Here's the drawing with two shaded views (mm, measured from the low corner). I have some questions. A direction names the side the tool comes from. Round coordinates to 2 decimals unless told otherwise and drop trailing zeros. Loops run counter-clockwise (first coordinate to the right, second up) from the corner with the lowest first, then second, coordinate; pieces in that order, holes last.
(1) I want a section at A-A on z = 10. Write out the boundary of the cut face in (x, y).
(2) If I drill on line 1 along Z through (x, y) = (15, 1.6); line 2 along Z through (x, y) = (2.2, 15); line 3 along Y through (x, z) = (14.5, 1.25), over which ranges is the centre line in solid material (lowest first)?
(3) Thinking about a two-plate mould opening in Y: for the marked faces 1, 2 and 3, which applies, released by +Y, released by -Y, zero draft, split by the parting line, or undercut?
(4) Will these pins go through, and if not, where does the flat tip stop? pin 1 Ø5 at (x, z) = (14, 2.5) entering from +Y; pin 2 Ø5 at (y, z) = (26.5, 6) entering from +X.
(5) I want a section at C-C on y = 15. Write out the boundary of the cut face in (x, z).
(6) I want a section at B-B on x = 15. Write out the boundary of the cut face in (y, z), plus the area to 3 significant figures.
(7) I want a section at D-D on z = 2.75. Write out the boundary of the cut face in (x, y), plus the area to 3 significant figures.
(8) Which directions (+Z, -Z, +X, -X, +Y, -Y) give clear straight access to the entire face, cutting with the end or side of a thin tool? Please do the marked faces 4 and 5.
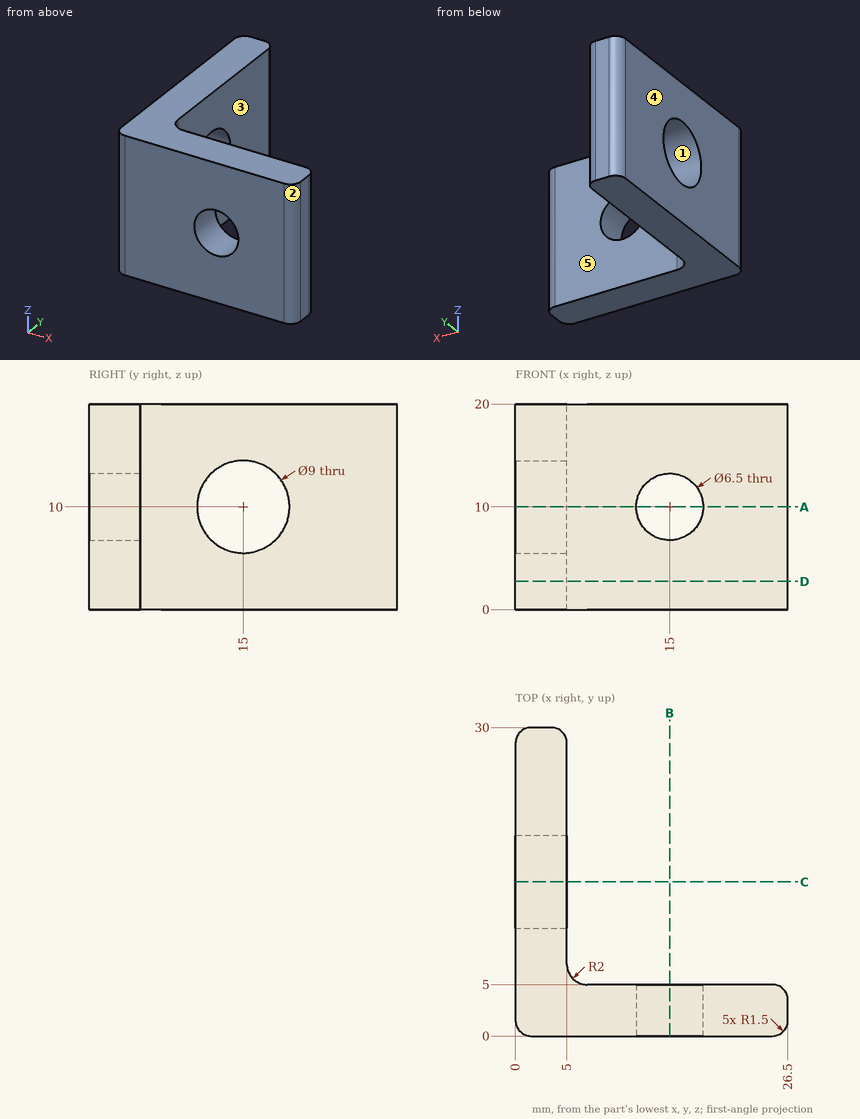
Filled sheet:
1. outline: (0, 1.5) arc R1.5 ccw to (1.5, 0) - (11.75, 0) - (11.75, 5) - (7, 5) arc R2 cw to (5, 7) - (5, 10.5) - (0, 10.5) - close; (0, 19.5) - (5, 19.5) - (5, 28.5) arc R1.5 ccw to (3.5, 30) - (1.5, 30) arc R1.5 ccw to (0, 28.5) - close; (18.25, 0) - (25, 0) arc R1.5 ccw to (26.5, 1.5) - (26.5, 3.5) arc R1.5 ccw to (25, 5) - (18.25, 5) - close
2. line 1: z = 0 to 6.75, 13.25 to 20
2. line 2: z = 0 to 5.5, 14.5 to 20
2. line 3: y = 0 to 5
3. face 1: undercut
3. face 2: released by -Y
3. face 3: zero draft
4. pin 1: stops at y = 5
4. pin 2: stops at x = 5
5. outline: (0, 0) - (5, 0) - (5, 5.5) - (0, 5.5) - close; (0, 14.5) - (5, 14.5) - (5, 20) - (0, 20) - close
6. outline: (0, 0) - (5, 0) - (5, 6.75) - (0, 6.75) - close; (0, 13.25) - (5, 13.25) - (5, 20) - (0, 20) - close
6. area: 67.5 mm2
7. outline: (0, 1.5) arc R1.5 ccw to (1.5, 0) - (25, 0) arc R1.5 ccw to (26.5, 1.5) - (26.5, 3.5) arc R1.5 ccw to (25, 5) - (7, 5) arc R2 cw to (5, 7) - (5, 28.5) arc R1.5 ccw to (3.5, 30) - (1.5, 30) arc R1.5 ccw to (0, 28.5) - close
7. area: 256 mm2
8. face 4: +Z, -Z, -X, +Y, -Y
8. face 5: +Z, -Z, +X, +Y
